Autodesk Inventor part; units mm, degrees
ref_plane "YZ Plane" through (0, 0, 0) normal (1, 0, 0) x (0, 1, 0)
ref_plane "XZ Plane" through (0, 0, 0) normal (0, 1, 0) x (-1, 0, 0)
ref_plane "XY Plane" through (0, 0, 0) normal (0, 0, 1) x (1, 0, 0)
sketch "スケッチ1" plane through (0, 0, 0) normal (0, 1, 0) x (-1, 0, 0)
  line L0 (4.6641, 14.0328) -> (-35.3359, 14.0328)
  line L1 (-35.3359, 14.0328) -> (-35.3359, -25.9672)
  line L2 (-35.3359, -25.9672) -> (4.6641, -25.9672)
  line L3 (4.6641, -25.9672) -> (4.6641, 14.0328)
  point P0 (0, 0)
  dimension "d0" = 40
  dimension "d1" = 40
extrude "押し出し1" add sketch "スケッチ1" along normal blind 20
sketch "スケッチ2" plane through (0, 20, 0) normal (0, 1, 0) x (1, 0, 0)
  line L0 (35.3359, 25.9672) -> (-4.6641, 25.9672)
  circle A0 centre (15.3359, 25.9672) radius 15
  line L1 (-4.6641, -14.0328) -> (35.3359, -14.0328)
  circle A1 centre (15.3359, -14.2518) radius 20.0012
  point P0 (0, 0)
  dimension "d4" = 30
hole "穴1" at (15.3359, 20, 14.2518) direction (0, -1, 0) diameter 40 depth 20
sketch "スケッチ3" plane through (0, 20, 0) normal (0, 1, 0) x (1, 0, 0)
  line L0 (35.3359, 25.9672) -> (-4.6641, 25.9672)
  circle A0 centre (15.3359, 25.9672) radius 15
  point P0 (0, 0)
  dimension "d12" = 30
hole "穴2" at (15.3359, 20, -25.9672) direction (0, -1, 0) diameter 30 depth 20
equation "\"BendRadius\" = Thickness"
equation "\"BendReliefWidth\" = Thickness"
equation "\"BendReliefDepth\" = 0.5 * Thickness"
equation "\"CornerReliefSize\" = 4 * Thickness"
equation "\"MinimumRemnant\" = 2 * Thickness"
equation "\"TransitionRadius\" = BendRadius"
equation "\"JacobiRadiusSize\" = BendRadius"
equation "\"GapSize\" = Thickness"
Here's how the part is built. I have some questions about the finished solid (model axes, mm). Coordinates: 2 decimals unless noted, no trailing zeros. Write each loop counter-clockwise with the first axis right and the second up, starting at its lowest first coordinate (ties: lowest second). Pieces come first, ordered by that corner, then holes. Notation, with made-up numbers: (-8, 72) - (13, 72) arc R20 cw to (13, 103) - close; hole circle Ø4 at (88, 72). An arc over 180 degrees is marked (long way). One line per item, written item: value.
1) I'm going to push flat-ended pins straight in: P1, Ø8, axis at x = 21.5, y = 17, coming from the -Z side; P2, Ø4, axis at x = 17.5, z = -10, coming from the -Y side; P3, Ø1, axis at x = 13.5, y = 11.5, coming from the +Z side; P4, Ø5, axis at x = 2.5, y = 14, coming from the +Z side. Where does each tip first touch, or does it pass through?
Model answer:
P1: stops at z = -14.94
P2: stops at y = 0
P3: stops at z = -5.61
P4: stops at z = 1.41
2) I need wall thicknesses on line 1 along Z through (x, y) = (15, 12.25); line 2 along X through (y, z) = (18.25, -12.5); line 3 along X through (y, z) = (1.25, 2.5). Which ranges of each line are inside material? Lowest first, please.
Model answer:
line 1: z = -10.97 to -5.75
line 2: x = -4.66 to 8.73, 21.94 to 35.34
line 3: x = -4.66 to -0.85, 31.52 to 35.34
3) We'd pull the mould along X, two halves only. Please class faces 1 (the flat face through (35.336, 10, -6)), 2 (the cylindrical face through (14.899, 9.86, -5.743)), 3 (the flat face through (33, 10, -25.967)): pulls with the +X half, pulls with the -X half, needs draft (parallel to the pull), parting line crosses it, or undercut.
Model answer:
face 1: pulls with the +X half
face 2: undercut
face 3: needs draft
4) Suppose I cut it at A-A on z = -12. Write out the boundary of the cut face in (x, y), and give its area (3 significant figures).
Model answer:
outline: (-4.66, 0) - (9.87, 0) - (9.87, 20) - (-4.66, 20) - close; (20.81, 0) - (35.34, 0) - (35.34, 20) - (20.81, 20) - close
area: 581 mm²
5) Suppose I cut it at C-C on z = -4. Write out the boundary of the cut face in (x, y).
Model answer:
outline: (-4.66, 0) - (7.16, 0) - (7.16, 20) - (-4.66, 20) - close; (23.51, 0) - (35.34, 0) - (35.34, 20) - (23.51, 20) - close
6) Suppose I cut it at D-D on x = 9.5. Write out the boundary of the cut face in (y, z), and give its area (3 significant figures).
Model answer:
outline: (0, -12.15) - (20, -12.15) - (20, -4.88) - (0, -4.88) - close
area: 145 mm²
